Source: CAD feature listing. Evaluate the final solid. Frame: model axes, mm. A direction names the side the tool comes from. Round coordinates to 2 decimals unless told otherwise and drop trailing zeros. Loops run counter-clockwise (first coordinate to the right, second up) from the corner with the lowest first, then second, coordinate; pieces in that order, holes last.
(1) Section C-C, the plane z = 34. Return the cut outline in (x, y).
(2) Mould query, pull axis X, two halves, no side actions, for faces 4 (the flat face through (23.458, -3, 78)), 5 (the flat face through (63.5, 1, 50)), 6 (the flat face through (-1, -63.5, 50)). Classes: pulls with the +X half, pulls with the -X half, needs draft (parallel to the pull), parting line crosses it, or undercut.
(3) Section B-B, the plane x = 35. Return the cut outline in (y, z).
(4) Section D-D, the plane y = 49.5. Return the cut outline in (x, z).
(5) Section A-A, the plane y = 6.5. Return the cut outline in (x, z).
(6) First-contact query: pin 1 Ø12.5 at (x, z) = (2.5, 24.5) entering from -Y. Flat tip, straight axial feed; report the tip coordinate or a pass-through.
(7) Set-up query: faces 1 (the flat face through (-12.916, -26, 19)), 2 (the cylindrical face through (-0.889, 31.773, 92.852)), 3 (the flat face through (-48.627, -57, 75)). Return all of +Z, -Z, +X, -X, +Y, -Y with unobstructed straight access to the full face (end or side cutting, diameter ignored); none if empty.
(8) Material intervals for probe 1 along X at (y, z) = (-44, 25.5); probe 2 along Z at (x, y) = (-21, -19.5); probe 3 along Z at (x, y) = (28.5, 44), sorted ascending.
```python
from build123d import *

# Parameters (mm, degrees)
F0_W     = 127
F0_H     = 127
F1_DEPTH = 101.6
F2_W     = 25.4
F2_H     = 38.1
F3_DEPTH = 76.2
F4_W     = 127
F4_H     = 127
F5_DEPTH = 2.54
F6_W     = 34.454562
F6_H     = 16.860753
F6_W_2   = 26.879448
F6_H_2   = 20.281769
F7_DEPTH = 127.001
F8_R     = 13.091888
F8_R_2   = 13.519639
F9_DEPTH = 127.001


with BuildPart() as f1:
    # F0 (on Top) → F1 (new body)
    with BuildSketch(Plane.XY):
        Rectangle(F0_W, F0_H)
    extrude(amount=F1_DEPTH)

    # F2 (on face) → F3 (cut)
    with BuildSketch(Plane.XZ.offset(63.5)):
        with Locations((-0.216101, 19.05)):
            Rectangle(F2_W, F2_H)
    extrude(amount=-F3_DEPTH, mode=Mode.SUBTRACT)

    # F4 (on face) → F5 (join)
    with BuildSketch(Plane(origin=(0, 0, 0), x_dir=(1, 0, 0), z_dir=(0, 0, -1))):
        Rectangle(F4_W, F4_H)
    extrude(amount=F5_DEPTH)

    # F6 (on face) → F7 (cut, through all)
    with BuildSketch(Plane(origin=(0, 63.5, 0), x_dir=(-1, 0, 0), z_dir=(0, 1, 0))):
        with Locations((31.400084, 74.889273)):
            Rectangle(F6_W, F6_H)
        with Locations((-36.898153, 78.310293)):
            Rectangle(F6_W_2, F6_H_2)
    extrude(amount=-F7_DEPTH, mode=Mode.SUBTRACT)

    # F8 (on face) → F9 (cut, through all)
    with BuildSketch(Plane(origin=(-63.5, 0, 0), x_dir=(0, -1, 0), z_dir=(-1, 0, 0))):
        with Locations((-30.068897, 79.871635)):
            Circle(F8_R)
        with Locations((38.37111, 79.601437)):
            Circle(F8_R_2)
    extrude(amount=-F9_DEPTH, mode=Mode.SUBTRACT)


solid = f1.part
```
Output values:
1. outline: (-63.5, -63.5) - (-12.92, -63.5) - (-12.92, 12.7) - (12.48, 12.7) - (12.48, -63.5) - (63.5, -63.5) - (63.5, 63.5) - (-63.5, 63.5) - close
2. face 4: undercut
2. face 5: pulls with the +X half
2. face 6: needs draft
3. outline: (-63.5, -2.54) - (63.5, -2.54) - (63.5, 68.17) - (35.94, 68.17) arc R13.09 cw to (24.2, 68.17) - (-31.15, 68.17) arc R13.52 cw to (-45.59, 68.17) - (-63.5, 68.17) - close; (-63.5, 88.45) - (-48.59, 88.45) arc R13.52 cw to (-28.15, 88.45) - (20.18, 88.45) arc R13.09 cw to (39.96, 88.45) - (63.5, 88.45) - (63.5, 101.6) - (-63.5, 101.6) - close
4. outline: (-63.5, -2.54) - (63.5, -2.54) - (63.5, 101.6) - (-63.5, 101.6) - close; hole (-48.63, 66.46) - (-14.17, 66.46) - (-14.17, 83.32) - (-48.63, 83.32) - close; hole (23.46, 68.17) - (50.34, 68.17) - (50.34, 88.45) - (23.46, 88.45) - close
5. outline: (-63.5, -2.54) - (63.5, -2.54) - (63.5, 101.6) - (-63.5, 101.6) - close; hole (-48.63, 66.46) - (-14.17, 66.46) - (-14.17, 83.32) - (-48.63, 83.32) - close; hole (-12.92, 0) - (12.48, 0) - (12.48, 38.1) - (-12.92, 38.1) - close; hole (23.46, 68.17) - (50.34, 68.17) - (50.34, 88.45) - (23.46, 88.45) - close
6. pin 1: stops at y = 12.7
7. face 1: -Y
7. face 2: +X, -X
7. face 3: +Y, -Y
8. probe 1: x = -63.5 to -12.92, 12.48 to 63.5
8. probe 2: z = -2.54 to 66.46, 83.32 to 101.6
8. probe 3: z = -2.54 to 68.17, 88.45 to 101.6
